Autodesk Fusion 360 part; units mm, degrees
sketch "Sketch1" plane through (0, 0, 0) normal (0, 0, 1) x (1, 0, 0)
  line L0 (3.81, 0) -> (13.716, 0)
  line L1 (13.716, 0) -> (13.716, 7.62)
  line L2 (13.716, 7.62) -> (3.81, 7.62)
  line L3 (0, 3.81) -> (0, 3.81)
  line L4 (6.096, 7.62) -> (6.096, 0)
  circle A0 centre (3.81, 3.81) radius 1.651
  arc A1 (0, 3.81) -> (3.81, 0) centre (3.81, 3.81) ccw
  arc A2 (3.81, 7.62) -> (0, 3.81) centre (3.81, 3.81) ccw
  point P0 (0, 7.62)
  dimension "d1" = 7.62
  dimension "d2" = 13.716
  dimension "d3" = 7.62
  dimension "d4" = 3.302
  dimension "d6" = 3.81
  dimension "d7" = 3.81
  dimension "d8" = 3.81
extrude "Extrude1" add sketch "Sketch1" along normal blind 3.302 contours L0 L2 L4 A1 A2
extrude "Extrude2" add sketch "Sketch1" along normal blind 2.286 contours L0 L1 L2 L4
Here's how the part is built. I have some questions about the finished solid (model axes, mm). A direction names the side the tool comes from. Round coordinates to 2 decimals unless told otherwise and drop trailing zeros. Loops run counter-clockwise (first coordinate to the right, second up) from the corner with the lowest first, then second, coordinate; pieces in that order, holes last. Notation, with made-up numbers: M 10.5,67.25 L 53.5,67.25 A10 cw 53.5,80.25 Z; hole C -3,22 d5. An arc over 180 degrees is marked long. Write each question's results on one line, items separated by ' | '. Start each with the question number.
(1) I want a section at C-C (y = 5). Please give me the cut outline in (x, z).
(2) Thinking about a two-plate mould opening in X: for faces 1 (the cylindrical face through (0, 3.7, 1.6)), 2 (the cylindrical face through (5.335, 4.442, 1.628)), 3 (the flat face through (7, 4, 0)), which applies, pulls with the +X half, pulls with the -X half, needs draft (parallel to the pull), parting line crosses it, or undercut?
(3) I want a section at B-B (z = 1.45). Please give me the cut outline in (x, y), then the cut area to 3 significant figures.
(4) I want a section at D-D (z = 2.5). Please give me the cut outline in (x, y), then the cut area to 3 significant figures.
(5) I want a section at A-A (y = 3.81). Please give me the cut outline in (x, z), then the cut area to 3 significant figures.
(6) Will this pin go through, and if not, where does the flat tip stop? P1, Ø2, axis at x = 3.81, y = 3.81, coming from the +Z side.
(7) If I drill on probe 1 along X at (y, z) = (3.75, 1); probe 2 along Y at (x, z) = (3.81, 1.85); probe 3 along Z at (x, y) = (10.5, 5), over which ranges is the centre line in solid material (lowest first)? Write a range as from..to.
(8) On a 3-axis mill with a long thin cutter (end or side, diameter ignored), from which of +Z, -Z, +X, -X, +Y, -Y can I reach the whole of each face in a straight line? I mean faces 4 (the flat face through (9, 7.62, 1)), 5 (the flat face through (6.096, 4, 3)). Say none if no direction works.
Solved:
1) outline: M 0.19,0 L 2.67,0 L 2.67,3.3 L 0.19,3.3 Z; M 4.95,0 L 13.72,0 L 13.72,2.29 L 6.1,2.29 L 6.1,3.3 L 4.95,3.3 Z
2) face 1: pulls with the -X half | face 2: undercut | face 3: needs draft
3) outline: M 3.81,0 L 13.72,0 L 13.72,7.62 L 3.81,7.62 A3.81 ccw Z; hole C 3.81,3.81 d3.3 | area: 89.7 mm²
4) outline: M 3.81,0 L 6.1,0 L 6.1,7.62 L 3.81,7.62 A3.81 ccw Z; hole C 3.81,3.81 d3.3 | area: 31.7 mm²
5) outline: M 0,0 L 2.16,0 L 2.16,3.3 L 0,3.3 Z; M 5.46,0 L 13.72,0 L 13.72,2.29 L 6.1,2.29 L 6.1,3.3 L 5.46,3.3 Z | area: 26.6 mm²
6) P1: passes through
7) probe 1: x = 0..2.16, 5.46..13.72 | probe 2: y = 0..2.16, 5.46..7.62 | probe 3: z = 0..2.29
8) face 4: +Z, -Z, +X, -X, +Y | face 5: +Z, +X, +Y, -Y
